Geometry check sheet. Reference: the model listing, model coordinates, mm. Coordinates: 2 decimals unless noted, no trailing zeros. Loops run counter-clockwise (first coordinate to the right, second up) from the corner with the lowest first, then second, coordinate; pieces in that order, holes last. Notation, with made-up numbers: (14, 63) -> (69, 63) arc R11 cw to (69, 71) -> close; hole circle Ø6 at (45.5, 58.25). An arc over 180 degrees is marked (long way). Answer as a JSON object with one key per item and string values.
from build123d import *

# Parameters (mm, degrees)
F0_W          = 100
F0_H          = 100
F1_DEPTH      = 50
F2_R          = 17.5
F3_DEPTH      = 50
F3_DEPTH_BACK = 110
F4_R          = 17.4779300175
F1_FACE1_W    = 100
F1_FACE1_H    = 100
F5_DEPTH      = 100.001


with BuildPart() as f1:
    # F0 (on Front) → F1 (new body, symmetric)
    with BuildSketch(Plane.XZ):
        with Locations((0, -2.4868422188)):
            Rectangle(F0_W, F0_H)
    extrude(amount=F1_DEPTH, both=True)

    # F2 (on Front) → F3 (cut, two sides)
    with BuildSketch(Plane.XZ) as f3_sk:
        Circle(F2_R)
    extrude(amount=F3_DEPTH, mode=Mode.SUBTRACT)
    extrude(f3_sk.sketch, amount=-F3_DEPTH_BACK, mode=Mode.SUBTRACT)

    # F4 (on face) + F1_face1 (on face) → F5 (cut, through all)
    with BuildSketch(Plane.YZ.offset(50)):
        Circle(F4_R)
    with BuildSketch(Plane(origin=(-50, 0, -2.4868422188), x_dir=(0, -1, 0), z_dir=(-1, 0, 0))):
        Rectangle(F1_FACE1_W, F1_FACE1_H)
    extrude(amount=-F5_DEPTH, dir=(1, 0, 0), mode=Mode.SUBTRACT)


solid = f1.part
1. Mould release check, pull along Y, two halves, no side actions. Record for faces 1 (the face through (-1, 50, 20)), 2 (the face through (-30.55, -17.46, 0.77)), 3 (the face through (8.075, -11.811, -15.526)): released by +Y, released by -Y, zero draft, split by the parting line, or undercut.
Evaluation:
{"face 1": "released by +Y", "face 2": "undercut", "face 3": "zero draft"}
2. Thickness scan on probe 1 along Y at (x, z) = (-31, 0); probe 2 along Z at (x, y) = (-32.5, 0); probe 3 along X at (y, z) = (-20, -9). Record the ranges inside material, lowest first. Write a range as from..to.
Evaluation:
{"probe 1": "y = -50..-17.48, 17.48..50", "probe 2": "z = -52.49..-17.48, 17.48..47.51", "probe 3": "x = -50..-15.01, 15.01..50"}
3. Section check D-D, the plane x = -8.5. Record the boundary of the cut face in (y, z), then the cut area to 3 significant figures.
Evaluation:
{"outline": "(-50, -52.49) -> (50, -52.49) -> (50, -15.3) -> (8.45, -15.3) arc R17.48 cw to (-8.45, -15.3) -> (-50, -15.3) -> close; (-50, 15.3) -> (-8.45, 15.3) arc R17.48 cw to (8.45, 15.3) -> (50, 15.3) -> (50, 47.51) -> (-50, 47.51) -> close", "area": "6,890 mm^2"}
4. Section check C-C, the plane z = 0. Record the boundary of the cut face in (x, y).
Evaluation:
{"outline": "(-50, -50) -> (-17.5, -50) -> (-17.5, -17.48) -> (-50, -17.48) -> close; (-50, 17.48) -> (-17.5, 17.48) -> (-17.5, 50) -> (-50, 50) -> close; (17.5, -50) -> (50, -50) -> (50, -17.48) -> (17.5, -17.48) -> close; (17.5, 17.48) -> (50, 17.48) -> (50, 50) -> (17.5, 50) -> close"}
5. Section check B-B, the plane x = -36.5. Record the boundary of the cut face in (y, z), then the cut area to 3 significant figures.
Evaluation:
{"outline": "(-50, -52.49) -> (50, -52.49) -> (50, 47.51) -> (-50, 47.51) -> close; hole circle Ø34.96 at (0, 0)", "area": "9,040 mm^2"}
6. Section check A-A, the plane y = 0. Record the boundary of the cut face in (x, z).
Evaluation:
{"outline": "(-50, -52.49) -> (50, -52.49) -> (50, -17.48) -> (0.88, -17.48) arc R17.5 cw to (-0.88, -17.48) -> (-50, -17.48) -> close; (-50, 17.48) -> (-0.88, 17.48) arc R17.5 cw to (0.88, 17.48) -> (50, 17.48) -> (50, 47.51) -> (-50, 47.51) -> close"}
